For this review, take the finished solid that the model builds, in its own axes (mm). A direction names the side the tool comes from. Give positions to 0.01 mm unless a question says otherwise; leave off trailing zeros. Loops run counter-clockwise (first coordinate to the right, second up) from the corner with the lowest first, then second, coordinate; pieces in that order, holes last.
```python
from build123d import *

# Parameters (mm, degrees)
SKETCH1_W           = 200
SKETCH1_H           = 200
SKETCH1_W_2         = 150
SKETCH1_H_2         = 150
BOSS_EXTRUDE1_DEPTH = 50
SKETCH2_W           = 170
SKETCH2_H           = 170
CUT_EXTRUDE1_DEPTH  = 22.5
FILLET1_R           = 4
FILLET2_R           = 4


with BuildPart() as part:
    # Sketch1 → Boss-Extrude1 (new, symmetric)
    with BuildSketch(Plane.XY):
        Rectangle(SKETCH1_W, SKETCH1_H)
        Rectangle(SKETCH1_W_2, SKETCH1_H_2, mode=Mode.SUBTRACT)
    extrude(amount=BOSS_EXTRUDE1_DEPTH, both=True)

    # Sketch2 → Cut-Extrude1 (cut, symmetric)
    with BuildSketch(Plane.XY):
        Rectangle(SKETCH2_W, SKETCH2_H)
    extrude(amount=CUT_EXTRUDE1_DEPTH, both=True, mode=Mode.SUBTRACT)

    # Fillet1
    fillet1_edges = [part.edges().sort_by_distance(p)[0] for p in [
        (0, -75, -22.5),
        (75, 0, -22.5),
        (0, 75, -22.5),
        (-75, 0, -22.5),
    ]]
    fillet(fillet1_edges, radius=FILLET1_R)

    # Fillet2
    fillet2_edges = [part.edges().sort_by_distance(p)[0] for p in [
        (0, -75, 22.5),
        (75, 0, 22.5),
        (0, 75, 22.5),
        (-75, 0, 22.5),
    ]]
    fillet(fillet2_edges, radius=FILLET2_R)


solid = part.part
```
Item 1: Clearance check with a flat-ended pin moving along its axis: pin 1 Ø12 at (x, y) = (-50.5, 65.5) entering from +Z. State where the tip first meets the part, or that it passes through.
Answer:
pin 1: passes through
Item 2: For L1, parallel to X at y = -27, z = -17; L2, parallel to Y at x = -10, z = -35, list the stretches that pass through material, from the lowest coordinate up.
Answer:
L1: x = -100 to -85, 85 to 100
L2: y = -100 to -75, 75 to 100
Item 3: Take a section at D-D on z = 11.5. Give the boundary of the cut face in (x, y).
Answer:
outline: (-100, -100) - (100, -100) - (100, 100) - (-100, 100) - close; hole (-85, -85) - (85, -85) - (85, 85) - (-85, 85) - close
Item 4: Tool access review of faces 4 (the flat face through (-1, -85, 0)), 5 (the flat face through (75, -1, -38)), 6 (the flat face through (-90, 1, 50)): name each direction out of +Z, -Z, +X, -X, +Y, -Y from which nothing blocks a thin tool from reaching the whole face with its end or side.
Answer:
face 4: none
face 5: +Z, -Z
face 6: +Z, +X, -X, +Y, -Y
Item 5: Take a section at A-A on x = 24.5. Give the boundary of the cut face in (y, z), and give its area (3 significant figures).
Answer:
outline: (-100, -50) - (-75, -50) - (-75, -26.5) arc R4 ccw to (-79, -22.5) - (-85, -22.5) - (-85, 22.5) - (-79, 22.5) arc R4 ccw to (-75, 26.5) - (-75, 50) - (-100, 50) - close; (75, -50) - (100, -50) - (100, 50) - (75, 50) - (75, 26.5) arc R4 ccw to (79, 22.5) - (85, 22.5) - (85, -22.5) - (79, -22.5) arc R4 ccw to (75, -26.5) - close
area: 4,090 mm2
Item 6: The part is to be moulded in two halves that separate along X. For faces 1 (the flat face through (-7, -81, -22.5)), 2 (the flat face through (-1, 100, 1)), 3 (the flat face through (100, -1, 1)), say which applies: released by +X, released by -X, zero draft, split by the parting line, or undercut.
Answer:
face 1: undercut
face 2: zero draft
face 3: released by +X
Item 7: Take a section at B-B on z = 38. Give the boundary of the cut face in (x, y).
Answer:
outline: (-100, -100) - (100, -100) - (100, 100) - (-100, 100) - close; hole (-75, -75) - (75, -75) - (75, 75) - (-75, 75) - close
